Here's the drawing with two shaded views (mm, measured from the low corner). I have some questions. Coordinates: 2 decimals unless noted, no trailing zeros. Write each loop counter-clockwise with the first axis right and the second up, starting at its lowest first coordinate (ties: lowest second). Pieces come first, ordered by that corner, then holes.
Item 1: I'm going to push flat-ended pins straight in: pin 1 Ø0.9 at (x, y) = (1.5, 38.5) entering from +Z; pin 2 Ø1.5 at (x, y) = (1, 24) entering from -Z; pin 3 Ø1.5 at (x, z) = (2, 1) entering from +Y. Where does each tip first touch, or does it pass through?
Item 2: If we section it at B-B (z = 19): Please give me the cut outline in (x, y).
Item 3: If we section it at A-A (y = 38.5): Please give me the cut outline in (x, z).
Item 4: If we section it at C-C (z = 26): Please give me the cut outline in (x, y).
Item 5: If I drill on line 1 (Z direction, x = 0.9, y = 25); line 2 (Z direction, x = 0.75, y = 17.5); line 3 (Y direction, x = 2.55, z = 25.5), over which ranges is the centre line in solid material (lowest first)?
Item 6: If we section it at D-D (z = 6): Please give me the cut outline in (x, y).
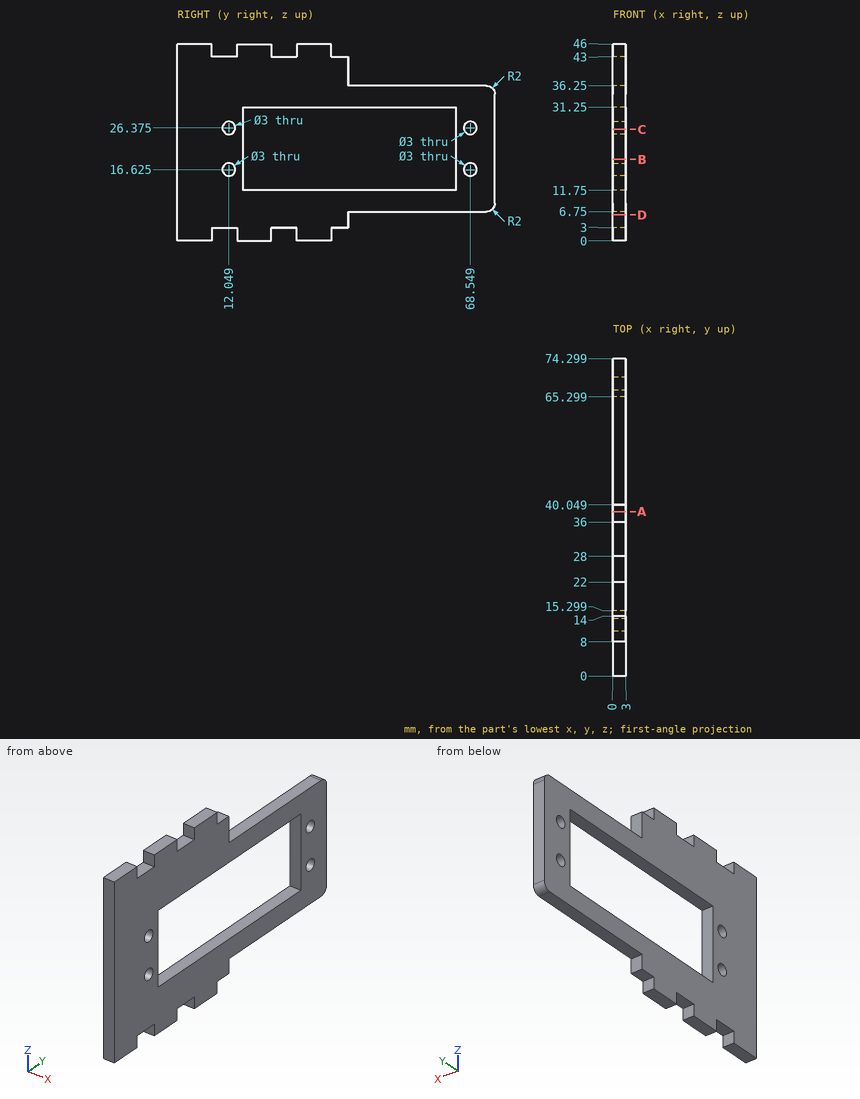
Answer list:
1. pin 1: stops at z = 43
1. pin 2: stops at z = 3
1. pin 3: stops at y = 36
2. outline: (0, 0) - (3, 0) - (3, 15.3) - (0, 15.3) - close; (0, 65.3) - (3, 65.3) - (3, 74.3) - (0, 74.3) - close
3. outline: (0, 3) - (3, 3) - (3, 11.75) - (0, 11.75) - close; (0, 31.25) - (3, 31.25) - (3, 43) - (0, 43) - close
4. outline: (0, 0) - (3, 0) - (3, 10.6) - (0, 10.6) - close; (0, 13.5) - (3, 13.5) - (3, 15.3) - (0, 15.3) - close; (0, 65.3) - (3, 65.3) - (3, 67.1) - (0, 67.1) - close; (0, 70) - (3, 70) - (3, 74.3) - (0, 74.3) - close
5. line 1: z = 3 to 11.75, 31.25 to 43
5. line 2: z = 0 to 11.75, 31.25 to 46
5. line 3: y = 0 to 10.83, 13.27 to 15.3, 65.3 to 67.33, 69.77 to 74.3
6. outline: (0, 0) - (3, 0) - (3, 40.05) - (0, 40.05) - close
